Geometry check sheet. Reference: the model listing, model coordinates, mm. A direction names the side the tool comes from. Round coordinates to 2 decimals unless told otherwise and drop trailing zeros. Loops run counter-clockwise (first coordinate to the right, second up) from the corner with the lowest first, then second, coordinate; pieces in that order, holes last. Notation, with made-up numbers: (-25.75, 87.5) -> (-7.75, 87.5) arc R15 ccw to (-7.75, 102.5) -> close; hole circle Ø9 at (46, 6). An arc over 180 degrees is marked (long way). Use a Markdown table: item, result. Add a question column.
Q1. Sectioned sample at D-D, the plane z = 3.5. Enter the section's corners in (x, y), then the cut area to 3 significant figures.
Q2. Release check for a two-part mould opening along X. For faces 1 (the face through (-7.938, 0, 2)), 2 (the face through (0, 0, 3.175)), 3 (the face through (0, -3.969, 2)), 4 (the face through (-4, 0, 3.175)) record: released by +X, released by -X, zero draft, split by the parting line, or undercut.
Q3. Set-up check for faces 5 (the face through (4.726, 0.238, 2.37)), 6 (the face through (6.24, 0.72, 3.96)), 7 (the face through (7.938, 0, 2)): record each of +Z, -Z, +X, -X, +Y, -Y from which the full face is reachable in a straight line by a thin tool's end or side.
Q4. Sectioned sample at B-B, the plane x = 0. Enter the section's corners in (y, z) (1 decimal), then the cut area to 3 significant figures.
Q5. Gauge pin test, flat ends, axial feed: P1, Ø1.4, axis at x = -3, y = -0.5, coming from the -Z side; P2, Ø2, axis at x = 0, y = 0, coming from the +Z side (3 decimals). Record the tip position at first contact, or that the pin passes through.
Q6. Material ranges on L1, parallel to X at y = 0, z = 2.55 (1 decimal); L2, parallel to X at y = 0, z = 0.75; L3, parallel to Y at x = 0, z = 0.95, recorded low to high.
Q7. Sectioned sample at A-A, the plane z = 2.7. Enter the section's corners in (x, y) (1 decimal), then the cut area to 3 significant figures.
```python
from build123d import *

# Parameters (mm, degrees)
F0_W     = 15.875
F0_H     = 7.9375
F0_R     = 2.38125
F1_DEPTH = 3.175
F2_DEPTH = 4.7625
F3_T     = -1.5875
F4_R     = 1.5875
F4_R_2   = 0.79375
F5_DEPTH = 1.5875


with BuildPart() as f1:
    # F0 (on Top) → F1 (new body)
    with BuildSketch(Plane.XY):
        Rectangle(F0_W, F0_H)
        with Locations((-3.96875, 0)):
            Circle(F0_R, mode=Mode.SUBTRACT)
        with Locations((3.96875, 0)):
            Circle(F0_R, mode=Mode.SUBTRACT)
    extrude(amount=F1_DEPTH)

    # F0 (on Top) → F2 (join)
    with BuildSketch(Plane.XY):
        with Locations((3.96875, 0)):
            Circle(F0_R)
        with Locations((-3.96875, 0)):
            Circle(F0_R)
    extrude(amount=F2_DEPTH)

    # F3
    f3_openings = [f1.faces().sort_by_distance(p)[0] for p in [
        (0, 0, 0),
    ]]
    offset(amount=F3_T, openings=f3_openings, kind=Kind.INTERSECTION)

    # F4 (on face) → F5 (join)
    with BuildSketch(Plane(origin=(0, 0, 1.5875), x_dir=(1, 0, 0), z_dir=(0, 0, -1))):
        Circle(F4_R)
        Circle(F4_R_2, mode=Mode.SUBTRACT)
    extrude(amount=F5_DEPTH)


solid = f1.part
```
Values:
| question | item | result |
|---|---|---|
| 1 | outline | circle Ø4.76 at (-3.97, 0); circle Ø4.76 at (3.97, 0) |
| 1 | area | 35.6 mm^2 |
| 2 | face 1 | released by -X |
| 2 | face 2 | undercut |
| 2 | face 3 | zero draft |
| 2 | face 4 | undercut |
| 3 | face 5 | -Z |
| 3 | face 6 | +Z |
| 3 | face 7 | +Z, -Z, +X, +Y, -Y |
| 4 | outline | (-4, 0) -> (-2.4, 0) -> (-2.4, 1.6) -> (-1.6, 1.6) -> (-1.6, 0) -> (-0.8, 0) -> (-0.8, 1.6) -> (0.8, 1.6) -> (0.8, 0) -> (1.6, 0) -> (1.6, 1.6) -> (2.4, 1.6) -> (2.4, 0) -> (4, 0) -> (4, 3.2) -> (-4, 3.2) -> close |
| 4 | area | 20.2 mm^2 |
| 5 | P1 | z = 1.59 |
| 5 | P2 | z = 3.175 |
| 6 | L1 | -7.9 to -4.8, -3.2 to 3.2, 4.8 to 7.9 |
| 6 | L2 | -7.94 to -6.35, -1.59 to -0.79, 0.79 to 1.59, 6.35 to 7.94 |
| 6 | L3 | -3.97 to -2.38, -1.59 to -0.79, 0.79 to 1.59, 2.38 to 3.97 |
| 7 | outline | (-7.9, -4) -> (7.9, -4) -> (7.9, 4) -> (-7.9, 4) -> close; hole circle Ø1.6 at (-4, 0); hole circle Ø1.6 at (4, 0) |
| 7 | area | 122 mm^2 |
